```python
from build123d import *

# Parameters (mm, degrees)
F0_W     = 598.5927433312
F0_H     = 341.3125
F0_R     = 2.15265
F0_R_2   = 1.7272
F0_W_2   = 41.275
F0_H_2   = 41.275
F1_DEPTH = 3.175
F3_R     = 4.7625
F2_R     = 1.7272
F4_DEPTH = 3.175
F5_R     = 1.7272
F6_DEPTH = 3.175


with BuildPart() as f1:
    # F0 (on Top) → F1 (new body)
    with BuildSketch(Plane.XY):
        with Locations((62.7588716656, 0)):
            Rectangle(F0_W, F0_H)
        with Locations((-128.6793928788, -62.7981428788)):
            Circle(F0_R, mode=Mode.SUBTRACT)
        with Locations((-119.1677433312, -63.3022737)):
            Circle(F0_R_2, mode=Mode.SUBTRACT)
        with Locations((119.1677433312, -63.3022737)):
            Circle(F0_R_2, mode=Mode.SUBTRACT)
        with Locations((178.6989933312, -72.23125)):
            Circle(F0_R_2, mode=Mode.SUBTRACT)
        with Locations((254.19713621, -62.7981428788)):
            Circle(F0_R, mode=Mode.SUBTRACT)
        with Locations((323.1614933312, -72.23125)):
            Circle(F0_R_2, mode=Mode.SUBTRACT)
        with Locations((-196.85, 72.23125)):
            Circle(F0_R_2, mode=Mode.SUBTRACT)
        with Locations((-128.6793928788, 62.7981428788)):
            Circle(F0_R, mode=Mode.SUBTRACT)
        with Locations((-119.1677433312, 63.3022737)):
            Circle(F0_R_2, mode=Mode.SUBTRACT)
        with Locations((-138.1125, 72.23125)):
            Circle(F0_R_2, mode=Mode.SUBTRACT)
        with Locations((-167.48125, 101.6)):
            Rectangle(F0_W_2, F0_H_2, mode=Mode.SUBTRACT)
        with Locations((-196.85, 130.96875)):
            Circle(F0_R_2, mode=Mode.SUBTRACT)
        with Locations((-138.1125, 130.96875)):
            Circle(F0_R_2, mode=Mode.SUBTRACT)
        with Locations((119.1677433312, 63.3022737)):
            Circle(F0_R_2, mode=Mode.SUBTRACT)
        with Locations((178.6989933312, 72.23125)):
            Circle(F0_R_2, mode=Mode.SUBTRACT)
        with Locations((254.19713621, 62.7981428788)):
            Circle(F0_R, mode=Mode.SUBTRACT)
        with Locations((323.1614933312, 72.23125)):
            Circle(F0_R_2, mode=Mode.SUBTRACT)
    extrude(amount=F1_DEPTH)

    # F3
    f3_edges = [f1.edges().sort_by_distance(p)[0] for p in [
        (362.055243, -170.65625, 1.5875),
        (-236.5375, -170.65625, 1.5875),
        (-236.5375, 170.65625, 1.5875),
        (362.055243, 170.65625, 1.5875),
    ]]
    fillet(f3_edges, radius=F3_R)

    # F2 (on face) → F4 (cut, through all)
    with BuildSketch(Plane.XY.offset(3.175)):
        with Locations((-206.375, -140.49375)):
            Circle(F2_R)
        with Locations((-206.375, 140.49375)):
            Circle(F2_R)
        with Locations((331.8927433312, 140.49375)):
            Circle(F2_R)
        with Locations((331.8927433312, -140.49375)):
            Circle(F2_R)
    extrude(amount=-F4_DEPTH, mode=Mode.SUBTRACT)

    # F5 (on face) → F6 (cut, through all)
    with BuildSketch(Plane.XY.offset(3.175)):
        with Locations((-134.9374857312, 0)):
            Circle(F5_R)
        with Locations((-204.7875, 0)):
            Circle(F5_R)
    extrude(amount=-F6_DEPTH, mode=Mode.SUBTRACT)


solid = f1.part
```
Can you work these out from the model? Positions are in its coordinate system, mm. Give positions to 0.01 mm unless a question says otherwise; leave off trailing zeros. Loops run counter-clockwise (first coordinate to the right, second up) from the corner with the lowest first, then second, coordinate; pieces in that order, holes last. Notation, with made-up numbers: M 79.5,59 L 134.5,59 A20 cw 134.5,73 Z; hole C -12.5,30 d10. An arc over 180 degrees is marked long. Answer in a Markdown table with one row per item.
1. Suppose I cut it at A-A on y = 102. Write out the boundary of the cut face in (x, z) (1 decimal).
Taken from the geometry:
| item | result |
|---|---|
| outline | M -236.5,0 L -188.1,0 L -188.1,3.2 L -236.5,3.2 Z; M -146.8,0 L 362.1,0 L 362.1,3.2 L -146.8,3.2 Z |
2. If I drill on line 1 along Y through (x, z) = (-168, 2.5); line 2 along X through (y, z) = (106, 0.75); line 3 along X through (y, z) = (-71.5, 1.4), over which ranges is the centre line in solid material (lowest first)?
Taken from the geometry:
| item | result |
|---|---|
| line 1 | y = -170.66 to 80.96, 122.24 to 170.66 |
| line 2 | x = -236.54 to -188.12, -146.84 to 362.06 |
| line 3 | x = -236.54 to 177.13, 180.26 to 321.6, 324.73 to 362.06 |
3. For pin 1 Ø3 at (x, y) = (178.7, 72.23) entering from +Z, with a flat end and sliding along its axis, tell me the tip position at first contact or that it passes through.
Taken from the geometry:
| item | result |
|---|---|
| pin 1 | passes through |
